```python
from build123d import *

# Parameters (mm, degrees)
SKETCH1_W                                = 65
SKETCH1_H                                = 80
BOSS_EXTRUDE1_DEPTH                      = 5
SKETCH2_W                                = 65
SKETCH2_H                                = 80
SKETCH2_W_2                              = 57
SKETCH2_H_2                              = 68
BOSS_EXTRUDE2_DEPTH                      = 30
SKETCH3_R                                = 3.85
BOSS_EXTRUDE3_DEPTH                      = 20
F_3_0MM_DOWEL_HOLE1_D                    = 3
F_3_0MM_DOWEL_HOLE1_DEPTH                = 8.5
F_3_0MM_DOWEL_HOLE1_CSINK_D              = 3.05
F_3_0MM_DOWEL_HOLE1_CSINK_ANGLE          = 90
F_3_0MM_DOWEL_HOLE1_TIP                  = 0.901290929
CUT_EXTRUDE1_DEPTH                       = 2.7
MIRROR1_AT_THE_SECOND_PLANE_COPY_1_DEPTH = 2.7
SKETCH13_R                               = 2.75
CUT_EXTRUDE4_DEPTH                       = 2.4
SKETCH14_R                               = 1.5
CUT_EXTRUDE5_DEPTH                       = 4
SKETCH11_W                               = 57
SKETCH11_H                               = 6
CUT_EXTRUDE2_DEPTH                       = 30
SKETCH15_W                               = 57
SKETCH15_H                               = 3.1
CUT_EXTRUDE6_DEPTH                       = 2.5
SKETCH16_W                               = 80
SKETCH16_H                               = 35
SKETCH16_R                               = 2.75
BOSS_EXTRUDE4_DEPTH                      = 2


with BuildPart() as part:
    # Sketch1 → Boss-Extrude1 (new body)
    with BuildSketch(Plane(origin=(0, 0, 0), x_dir=(1, 0, 0), z_dir=(0, 1, 0))):
        Rectangle(SKETCH1_W, SKETCH1_H)
    extrude(amount=BOSS_EXTRUDE1_DEPTH)

    # Sketch2 → Boss-Extrude2 (add)
    with BuildSketch(Plane(origin=(0, 5, 0), x_dir=(1, 0, 0), z_dir=(0, 1, 0))):
        Rectangle(SKETCH2_W, SKETCH2_H)
        Rectangle(SKETCH2_W_2, SKETCH2_H_2, mode=Mode.SUBTRACT)
    extrude(amount=BOSS_EXTRUDE2_DEPTH)

    # Sketch3 → Boss-Extrude3 (add)
    with BuildSketch(Plane(origin=(0, 5, 0), x_dir=(1, 0, 0), z_dir=(0, 1, 0))):
        with Locations(Location((-20.5, -28, 0), (0, 0, 90))):
            Circle(SKETCH3_R)
        with Locations(Location((20.5, -28, 0), (0, 0, 90))):
            Circle(SKETCH3_R)
        with Locations(Location((20.5, 28, 0), (0, 0, 90))):
            Circle(SKETCH3_R)
        with Locations(Location((-20.5, 28, 0), (0, 0, 90))):
            Circle(SKETCH3_R)
    extrude(amount=BOSS_EXTRUDE3_DEPTH)

    # Ø3.0mm Dowel Hole1
    with Locations(Plane(origin=(0, 25, 0), x_dir=(1, 0, 0), z_dir=(0, 1, 0))):
        with Locations((-20.5, 28), (20.5, 28), (20.5, -28), (-20.5, -28)):
            CounterSinkHole(F_3_0MM_DOWEL_HOLE1_D / 2, F_3_0MM_DOWEL_HOLE1_CSINK_D / 2, depth=F_3_0MM_DOWEL_HOLE1_DEPTH, counter_sink_angle=F_3_0MM_DOWEL_HOLE1_CSINK_ANGLE)
            with Locations((0, 0, -(F_3_0MM_DOWEL_HOLE1_DEPTH + F_3_0MM_DOWEL_HOLE1_TIP / 2))):  # 118° drill point
                Cone(0, F_3_0MM_DOWEL_HOLE1_D / 2, F_3_0MM_DOWEL_HOLE1_TIP, mode=Mode.SUBTRACT)

    # Sketch8 → Cut-Extrude1 (cut)
    with BuildSketch(Plane(origin=(0, 25, 0), x_dir=(1, 0, 0), z_dir=(0, 1, 0))):
        Polygon((-17.382308546, 28), (-18.941154273, 30.7), (-22.058845727, 30.7), (-23.617691454, 28), (-22.058845727, 25.3), (-18.941154273, 25.3), align=None)
    cut_extrude1 = extrude(amount=-CUT_EXTRUDE1_DEPTH, mode=Mode.SUBTRACT)

    # Mirror1: Cut-Extrude1 across plane
    add(cut_extrude1.mirror(Plane.XY), mode=Mode.SUBTRACT)

    # Mirror1 at the second plane: Cut-Extrude1 across plane
    add(cut_extrude1.mirror(Plane(origin=(0, 0, 0), x_dir=(0, 0, 1), z_dir=(1, 0, 0))), mode=Mode.SUBTRACT)

    # Mirror1 at the second plane copy 1 sketc → Mirror1 at the second plane copy 1 (cut)
    with BuildSketch(Plane(origin=(0, 25, 0), x_dir=(-1, 0, 0), z_dir=(0, 1, 0))):
        Polygon((-17.382308546, 28), (-18.941154273, 30.7), (-22.058845727, 30.7), (-23.617691454, 28), (-22.058845727, 25.3), (-18.941154273, 25.3), align=None)
    extrude(amount=-MIRROR1_AT_THE_SECOND_PLANE_COPY_1_DEPTH, mode=Mode.SUBTRACT)

    # Sketch13 → Cut-Extrude4 (cut)
    with BuildSketch(Plane(origin=(32.5, 0, 0), x_dir=(0, 0, -1), z_dir=(1, 0, 0))):
        with Locations((-36.6, 17.5)):
            Circle(SKETCH13_R)
    cut_extrude4 = extrude(amount=-CUT_EXTRUDE4_DEPTH, mode=Mode.SUBTRACT)

    # Sketch14 → Cut-Extrude5 (cut)
    with BuildSketch(Plane(origin=(32.5, 0, 0), x_dir=(0, 0, -1), z_dir=(1, 0, 0))):
        with Locations((-36.6, 17.5)):
            Circle(SKETCH14_R)
    cut_extrude5 = extrude(amount=-CUT_EXTRUDE5_DEPTH, mode=Mode.SUBTRACT)

    # Mirror2: Cut-Extrude4, Cut-Extrude5 across plane
    add(cut_extrude4.mirror(Plane(origin=(0, 0, 0), x_dir=(0, 0, 1), z_dir=(1, 0, 0))), mode=Mode.SUBTRACT)
    add(cut_extrude5.mirror(Plane(origin=(0, 0, 0), x_dir=(0, 0, 1), z_dir=(1, 0, 0))), mode=Mode.SUBTRACT)

    # Sketch11 → Cut-Extrude2 (cut)
    with BuildSketch(Plane(origin=(0, 35, 0), x_dir=(1, 0, 0), z_dir=(0, 1, 0))):
        with Locations((0, -37)):
            Rectangle(SKETCH11_W, SKETCH11_H)
    extrude(amount=-CUT_EXTRUDE2_DEPTH, mode=Mode.SUBTRACT)

    # Sketch15 → Cut-Extrude6 (cut)
    with BuildSketch(Plane(origin=(0, 5, 0), x_dir=(1, 0, 0), z_dir=(0, 1, 0))):
        with Locations((0, -35.55)):
            Rectangle(SKETCH15_W, SKETCH15_H)
    extrude(amount=-CUT_EXTRUDE6_DEPTH, mode=Mode.SUBTRACT)

    # Sketch16 → Boss-Extrude4 (add)
    with BuildSketch(Plane.ZY.offset(32.5)):
        with Locations((0, 17.5)):
            Rectangle(SKETCH16_W, SKETCH16_H)
        with Locations(Location((36.6, 17.5, 0), (0, 0, 180))):
            Circle(SKETCH16_R, mode=Mode.SUBTRACT)
    boss_extrude4 = extrude(amount=BOSS_EXTRUDE4_DEPTH)

    # Mirror3: Boss-Extrude4 across plane
    add(boss_extrude4.mirror(Plane(origin=(0, 0, 0), x_dir=(0, 0, 1), z_dir=(1, 0, 0))))


solid = part.part
```
Input: part model. Units: mm. Frame: model coordinates. A direction names the side the tool comes from. Coordinates: 2 decimals unless noted, no trailing zeros. Order: outer loops, then holes, each group sorted by start corner. A loop starts at its lowest first (then second) coordinate and runs counter-clockwise, first axis right, second up. Notation, with made-up numbers: (6, 7) - (34, 7) arc R13 ccw to (34, 31) - close; hole circle Ø9 at (75.25, -2). An arc over 180 degrees is marked (long way). Put each result on its own line as item: value.
1. Reachability of faces 4 (the face through (0, 17, -40)), 5 (the face through (-17.67, 25, -28.84)), 6 (the face through (-19.39, 19.36, 26.99)) from +Z, -Z, +X, -X, +Y, -Y: full face, straight path, thin tool, end or side. Return the list, or none.
Report:
face 4: -Z, +X, -X, +Y, -Y
face 5: +Z, +Y
face 6: +Y
2. Cut plane B-B on x = -15.5. Return the cut outline in (y, z).
Report:
outline: (0, -40) - (35, -40) - (35, -34) - (5, -34) - (5, 34) - (2.5, 34) - (2.5, 37.1) - (5, 37.1) - (5, 40) - (0, 40) - close
3. Contact query for flat-ended pins moving along their axis: pin 1 Ø1 at (x, y) = (-7.5, 28.5) entering from +Z; pin 2 Ø12 at (x, y) = (0.5, 6) entering from +Z; pin 3 Ø1.5 at (x, z) = (-2, 8) entering from +Y; pin 4 Ø3 at (y, z) = (18, 36) entering from +X. Output: stop coordinate, or through.
Report:
pin 1: stops at z = -34
pin 2: stops at z = 40
pin 3: stops at y = 5
pin 4: stops at x = 30.1
4. Cut plane A-A on y = 8.5. Return the cut outline in (x, z).
Report:
outline: (-34.5, -40) - (34.5, -40) - (34.5, 40) - (28.5, 40) - (28.5, -34) - (-28.5, -34) - (-28.5, 40) - (-34.5, 40) - close; circle Ø7.7 at (-20.5, -28); circle Ø7.7 at (-20.5, 28); circle Ø7.7 at (20.5, -28); circle Ø7.7 at (20.5, 28)
5. Cut plane C-C on y = 26.5. Return the cut outline in (x, z).
Report:
outline: (-34.5, -40) - (34.5, -40) - (34.5, 40) - (28.5, 40) - (28.5, -34) - (-28.5, -34) - (-28.5, 40) - (-34.5, 40) - close
6. Cut plane D-D on z = 1. Return the cut outline in (x, y).
Report:
outline: (-34.5, 0) - (34.5, 0) - (34.5, 35) - (28.5, 35) - (28.5, 5) - (-28.5, 5) - (-28.5, 35) - (-34.5, 35) - close
7. Line query: line 1 along X through (y, z) = (20.4, 28); line 2 along Z through (x, y) = (20.5, 23); line 3 along Z through (x, y) = (-20.5, 19). Output: solid intervals per line, ascending.
Report:
line 1: x = -34.5 to -28.5, -24.35 to -22, -19 to -16.65, 16.65 to 19, 22 to 24.35, 28.5 to 34.5
line 2: z = -40 to -34, -31.85 to -30.7, -25.3 to -24.15, 24.15 to 25.3, 30.7 to 31.85
line 3: z = -40 to -34, -31.85 to -29.5, -26.5 to -24.15, 24.15 to 26.5, 29.5 to 31.85
8. Draft query along X for faces 1 (the face through (34.5, 18, -1)), 2 (the face through (2, 35, -36)), 3 (the face through (-20.259, 15.755, 28.1)). Return one class per face: pulls with the +X half, pulls with the -X half, needs draft (parallel to the pull), parting line crosses it, or undercut.
Report:
face 1: pulls with the +X half
face 2: needs draft
face 3: undercut
